Source: three-view drawing plus pictorial views. Frame: mm from the lowest corner of the part. Round coordinates to 2 decimals unless told otherwise and drop trailing zeros. Order: outer loops, then holes, each group sorted by start corner. A loop starts at its lowest first (then second) coordinate and runs counter-clockwise, first axis right, second up. Notation, with made-up numbers: (-26.75, -26.5) -> (26.25, -26.5) arc R26 ccw to (26.25, 7.5) -> close; hole circle Ø11 at (87.25, 81.25). An arc over 180 degrees is marked (long way). Use a Markdown table: item, result.
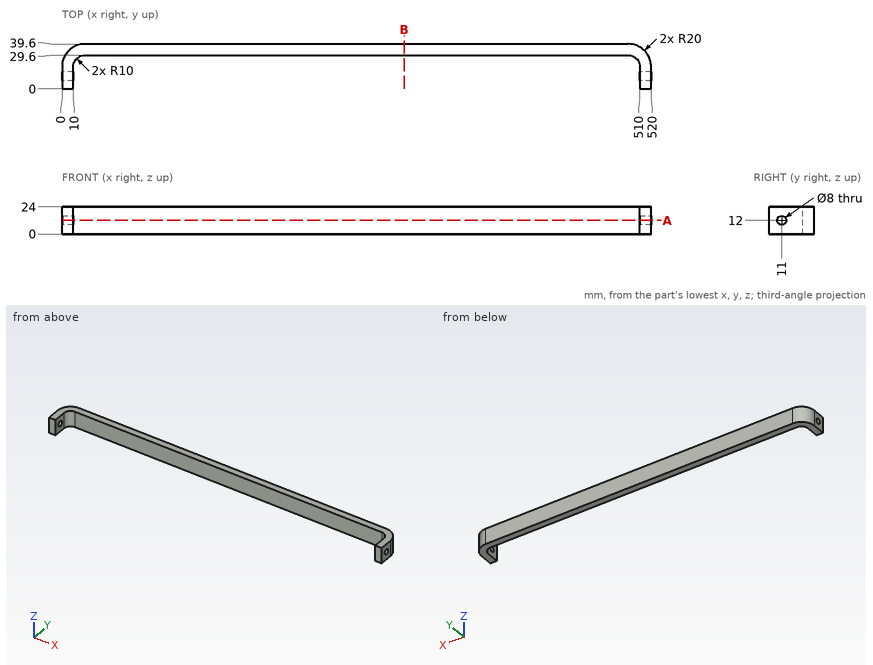
1) Line query: L1, parallel to X at y = 21, z = 8.75; L2, parallel to X at y = 12.5, z = 18.75; L3, parallel to Y at x = 163.5, z = 18. Output: solid intervals per line, ascending. Write a range as [from, to].
Results found:
| item | result |
|---|---|
| L1 | x = [0.05, 10.1], [509.9, 519.95] |
| L2 | x = [0, 10], [510, 520] |
| L3 | y = [29.6, 39.6] |
2) Cut plane B-B on x = 302. Return loops of the section in (y, z), and give its area (3 significant figures).
Results found:
| item | result |
|---|---|
| outline | (29.6, 0) -> (39.6, 0) -> (39.6, 24) -> (29.6, 24) -> close |
| area | 240 mm² |
3) Pin query (flat end, axial travel): pin 1 Ø2 at (x, z) = (158.5, 18) entering from -Y; pin 2 Ø10.5 at (y, z) = (11, 12) entering from +X. Return the tip coordinate at first contact, or that it passes through.
Results found:
| item | result |
|---|---|
| pin 1 | stops at y = 29.6 |
| pin 2 | stops at x = 520 |
4) Cut plane A-A on z = 12. Return loops of the section in (x, y).
Results found:
| item | result |
|---|---|
| outline | (0, 0) -> (10, 0) -> (10, 7) -> (0, 7) -> close; (0, 15) -> (10, 15) -> (10, 19.6) arc R10 cw to (20, 29.6) -> (500, 29.6) arc R10 cw to (510, 19.6) -> (510, 15) -> (520, 15) -> (520, 19.6) arc R20 ccw to (500, 39.6) -> (20, 39.6) arc R20 ccw to (0, 19.6) -> close; (510, 0) -> (520, 0) -> (520, 7) -> (510, 7) -> close |
